Read the model definition and answer for the solid it produces. Units are mm, in the model's axes. A direction names the side the tool comes from. Round coordinates to 2 decimals unless told otherwise and drop trailing zeros. Loops run counter-clockwise (first coordinate to the right, second up) from the corner with the lowest first, then second, coordinate; pieces in that order, holes last. Notation, with made-up numbers: M 55,7 L 111,7 A11 ccw 111,24 Z; hole C 54.5,-7 d9. An arc over 180 degrees is marked long. Write each question's results on one line, items separated by ' | '.
from build123d import *

# Parameters (mm, degrees)
DODANIE_WYCI_GNI_CIE1_DEPTH = 6


with BuildPart() as part:
    # Szkic2 → Dodanie-wyciągnięcie1 (new body)
    with BuildSketch(Plane.XY):
        with BuildLine():
            Line((5, 93.695492388), (11.889307623, 93.695492388))
            ThreePointArc((11.889307623, 93.695492388), (16.836926807, 89.417340299), (13.317879052, 83.903918151))
            ThreePointArc((13.317879052, 83.903918151), (12.285740172, 83.182517065), (11.889307623, 81.987288456))
            Line((11.889307623, 81.987288456), (11.889307623, 59.797095598))
            ThreePointArc((11.889307623, 59.797095598), (10.717734748, 56.968668473), (7.889307623, 55.797095598))
            Line((7.889307623, 55.797095598), (0, 55.797095598))
            Line((0, 55.797095598), (0, 63.247095598))
            Line((0, 63.247095598), (3, 63.247095598))
            Line((3, 63.247095598), (3, 61.872095598))
            Line((3, 61.872095598), (5, 61.872095598))
            Line((5, 61.872095598), (5, 63.247095598))
            Line((5, 63.247095598), (6, 63.247095598))
            Line((6, 63.247095598), (6, 66.347095598))
            Line((6, 66.347095598), (5, 66.347095598))
            Line((5, 66.347095598), (5, 67.722095598))
            Line((5, 67.722095598), (3, 67.722095598))
            Line((3, 67.722095598), (3, 66.347095598))
            Line((3, 66.347095598), (0, 66.347095598))
            Line((0, 66.347095598), (0, 74.247095598))
            Line((0, 74.247095598), (3, 74.247095598))
            Line((3, 74.247095598), (3, 72.872095598))
            Line((3, 72.872095598), (5, 72.872095598))
            Line((5, 72.872095598), (5, 74.247095598))
            Line((5, 74.247095598), (6, 74.247095598))
            Line((6, 74.247095598), (6, 77.245492388))
            Line((6, 77.245492388), (5, 77.245492388))
            Line((5, 77.245492388), (5, 78.620492388))
            Line((5, 78.620492388), (3, 78.620492388))
            Line((3, 78.620492388), (3, 77.245492388))
            Line((3, 77.245492388), (0, 77.245492388))
            Line((0, 77.245492388), (0, 88.695492388))
            ThreePointArc((0, 88.695492388), (1.464466094, 92.231026294), (5, 93.695492388))
        make_face()
    extrude(amount=-DODANIE_WYCI_GNI_CIE1_DEPTH)


solid = part.part
Item 1: For faces 1 (the face through (3, 74, -3)), 2 (the face through (7, 75, -6)), 3 (the face through (6, 76, -3)), determine the directions among +Z, -Z, +X, -X, +Y, -Y from which every point of the face is accessible in a straight line to the end or side of a thin tool.
Outcome:
face 1: +Z, -Z | face 2: -Z, +X, -X, +Y, -Y | face 3: +Z, -Z, -X
Item 2: Straight lines are drawn through the part: line 1 (Y direction, x = 2.5, z = -3.75); line 2 (X direction, y = 78, z = -4.2); line 3 (X direction, y = 65, z = -5.2). For each, find the intervals that lie inside material, in ascending order.
Outcome:
line 1: y = 55.8 to 63.25, 66.35 to 74.25, 77.25 to 93.03 | line 2: x = 0 to 3, 5 to 11.89 | line 3: x = 6 to 11.89
Item 3: The mould has two halves that part along X. Classify faces 4 (the face through (1, 63.247, -3)), 5 (the face through (16.82, 89.52, -2.96)), 6 (the face through (5, 78, -3)): pulls with the +X half, pulls with the -X half, needs draft (parallel to the pull), parting line crosses it, or undercut.
Outcome:
face 4: needs draft | face 5: pulls with the +X half | face 6: undercut
Item 4: The part is cut by section C-C (y = 79). Determine the outline of the cut face in (x, z), plus the area to 3 significant figures.
Outcome:
outline: M 0,-6 L 11.89,-6 L 11.89,0 L 0,0 Z | area: 71.3 mm2
Item 5: The part is cut by section D-D (x = 12.25). Determine the outline of the cut face in (y, z).
Outcome:
outline: M 83.13,-6 L 93.68,-6 L 93.68,0 L 83.13,0 Z
Item 6: The part is cut by section B-B (x = 1). Determine the outline of the cut face in (y, z).
Outcome:
outline: M 55.8,-6 L 63.25,-6 L 63.25,0 L 55.8,0 Z; M 66.35,-6 L 74.25,-6 L 74.25,0 L 66.35,0 Z; M 77.25,-6 L 91.7,-6 L 91.7,0 L 77.25,0 Z
Item 7: Flat-ended cylindrical pins translate along their axes: pin 1 (0.9 mm diameter, centred on y = 65.5, z = -4, fed in from -X); pin 2 (2.5 mm diameter, centred on x = 2, z = -3, fed in from +Y); pin 3 (1.5 mm diameter, centred on y = 67.5, z = -1.5, fed in from +X). Find the tip coordinate at first contact, or state that the pin passes through.
Outcome:
pin 1: stops at x = 6 | pin 2: stops at y = 93.38 | pin 3: stops at x = 11.89
